```python
from build123d import *

# Parameters (mm, degrees)
BOSS_EXTRUDE1_DEPTH      = 11.85
BOSS_EXTRUDE2_DEPTH      = 2
BOSS_EXTRUDE2_DEPTH_BACK = 13.85
SKETCH2_W                = 7
SKETCH2_H                = 1.8
FILLET1_R                = 6
CUT_EXTRUDE1_DEPTH       = 0.5
CUT_EXTRUDE2_DEPTH       = 0.5
SKETCH6_R                = 2.65
SKETCH6_R_2              = 1.5
CUT_EXTRUDE3_DEPTH       = 10


with BuildPart() as part:
    # Sketch1 → Boss-Extrude1 (new body)
    with BuildSketch(Plane.XY):
        with BuildLine():
            Line((-40, 25.458108108), (-17.056531053, 25.458108108))
            ThreePointArc((-17.056531053, 25.458108108), (-18.352562381, 15.292302634), (-15, 5.608108108))
            Line((-15, 5.608108108), (-40, 5.608108108))
            Line((-40, 5.608108108), (-40, 25.458108108))
        make_face()
    extrude(amount=BOSS_EXTRUDE1_DEPTH)

    # Sketch2 → Boss-Extrude2 (add, two sides: drawn at the far end of the back side and taken through both)
    with BuildSketch(Plane(origin=(0, 0, 0), x_dir=(-1, 0, 0), z_dir=(0, 0, -1)).offset(-BOSS_EXTRUDE2_DEPTH_BACK)):
        with Locations((36.5, 6.508108108)):
            Rectangle(SKETCH2_W, SKETCH2_H)
        with Locations((36.5, 24.558108108)):
            Rectangle(SKETCH2_W, SKETCH2_H)
    extrude(amount=BOSS_EXTRUDE2_DEPTH + BOSS_EXTRUDE2_DEPTH_BACK)

    # Fillet1
    # the kernel refuses this fillet: 6 mm, written as the material it takes off along each edge
    with BuildSketch(Plane(origin=(4, 17.608108108, 0), x_dir=(-0.5195868737353421, 0.854417626598336, 0), z_dir=(0.854417626598336, 0.5195868737353421, 0))) as fillet1_piece_1:
        with BuildLine():
            CenterArc((22.472205054 + FILLET1_R, FILLET1_R), FILLET1_R, 180, 90)
            Line((22.472205054 + FILLET1_R, 0), (22.472205054, 0))
            Line((22.472205054, 0), (22.472205054, FILLET1_R))
        make_face()
    revolve(axis=Axis((4, 17.608108108, 0), (0, 0, 1)), revolution_arc=129.220802233, mode=Mode.SUBTRACT)
    with BuildSketch(Plane(origin=(4, 17.608108108, 11.85), x_dir=(-0.5195868737353421, 0.854417626598336, 0), z_dir=(0.854417626598336, 0.5195868737353421, 0))) as fillet1_piece_2:
        with BuildLine():
            CenterArc((22.472205054 + FILLET1_R, -FILLET1_R), FILLET1_R, 90, 90)
            Line((22.472205054, -FILLET1_R), (22.472205054, 0))
            Line((22.472205054, 0), (22.472205054 + FILLET1_R, 0))
        make_face()
    revolve(axis=Axis((4, 17.608108108, 11.85), (0, 0, 1)), revolution_arc=129.220802233, mode=Mode.SUBTRACT)

    # Sketch3 → Cut-Extrude1 (cut)
    with BuildSketch(Plane(origin=(0, 25.458108108, 0), x_dir=(1, 0, 0), z_dir=(0, 1, 0))):
        with BuildLine():
            Line((-40, -0.925), (-22.180241126, -0.925))
            add(Edge.make_bspline(
                [(-18.937526934, -2.925), (-19.013227922, -2.828512493), (-19.092514949, -2.73433601), (-19.290739716, -2.514692345), (-19.412819443, -2.391961398), (-19.796517456, -2.041181837), (-20.076726357, -1.829898628), (-20.674341708, -1.461904013), (-20.986869841, -1.307747212), (-21.591258811, -1.074971042), (-21.88385471, -0.988046248), (-22.180241126, -0.925)],
                knots=[0.393521627, 0.393521627, 0.393521627, 0.393521627, 0.4375, 0.4375, 0.5, 0.5, 0.625, 0.625, 0.75, 0.75, 0.857744944, 0.857744944, 0.857744944, 0.857744944], degree=3))
            Line((-18.937526934, -2.925), (-40, -2.925))
            Line((-40, -2.925), (-40, -0.925))
        make_face()
        with BuildLine():
            Line((-40, -4.925), (-17.97760602, -4.925))
            add(Edge.make_bspline(
                [(-17.857114262, -5.924996789), (-17.862389732, -5.585330665), (-17.903230985, -5.251628442), (-17.97760602, -4.925)],
                knots=[0, 0, 0, 0, 0.123073848, 0.123073848, 0.123073848, 0.123073848], degree=3))
            add(Edge.make_bspline(
                [(-17.977607618, -6.925), (-17.903108355, -6.597642735), (-17.862351336, -6.26181668), (-17.857114262, -5.924996789)],
                knots=[0.87810057, 0.87810057, 0.87810057, 0.87810057, 1, 1, 1, 1], degree=3))
            Line((-17.977607618, -6.925), (-40, -6.925))
            Line((-40, -6.925), (-40, -4.925))
        make_face()
        with BuildLine():
            Line((-40, -8.925), (-18.937485208, -8.925))
            add(Edge.make_bspline(
                [(-22.180090087, -10.925), (-22.058031588, -10.899076779), (-21.936790659, -10.869159263), (-21.647506804, -10.787627729), (-21.479286663, -10.731759415), (-20.988005272, -10.542973422), (-20.675799804, -10.388674568), (-20.230975304, -10.115240101), (-20.087143687, -10.017400974), (-19.80724707, -9.806950573), (-19.671333831, -9.694234428), (-19.322525279, -9.375728013), (-19.120509969, -9.15842179), (-18.937485208, -8.925)],
                knots=[0.142746843, 0.142746843, 0.142746843, 0.142746843, 0.1875, 0.1875, 0.25, 0.25, 0.375, 0.375, 0.4375, 0.4375, 0.5, 0.5, 0.607411447, 0.607411447, 0.607411447, 0.607411447], degree=3))
            Line((-22.180090087, -10.925), (-40, -10.925))
            Line((-40, -10.925), (-40, -8.925))
        make_face()
    extrude(amount=-CUT_EXTRUDE1_DEPTH, mode=Mode.SUBTRACT)

    # Sketch4 → Cut-Extrude2 (cut)
    with BuildSketch(Plane.XZ.offset(-5.608108108)):
        with BuildLine():
            Line((-18.937485208, 8.925), (-40, 8.925))
            Line((-40, 8.925), (-40, 10.925))
            Line((-40, 10.925), (-22.180090087, 10.925))
            add(Edge.make_bspline(
                [(-22.180090087, 10.925), (-22.058031589, 10.899076779), (-21.936790659, 10.869159263), (-21.647506804, 10.787627729), (-21.479286663, 10.731759415), (-20.988005272, 10.542973422), (-20.675799804, 10.388674568), (-20.230975304, 10.115240101), (-20.087143687, 10.017400974), (-19.80724707, 9.806950573), (-19.671333831, 9.694234428), (-19.322525301, 9.375728033), (-19.12051001, 9.158421833), (-18.937485208, 8.925)],
                knots=[0.392588564, 0.392588564, 0.392588564, 0.392588564, 0.437341721, 0.437341721, 0.499841721, 0.499841721, 0.624841721, 0.624841721, 0.687341721, 0.687341721, 0.749841721, 0.749841721, 0.857253157, 0.857253157, 0.857253157, 0.857253157], degree=3))
        make_face()
        with BuildLine():
            Line((-40, 6.925), (-17.977607618, 6.925))
            add(Edge.make_bspline(
                [(-17.977607618, 6.925), (-17.903108355, 6.597642735), (-17.862351336, 6.26181668), (-17.857114262, 5.924996789)],
                knots=[0, 0, 0, 0, 0.12189943, 0.12189943, 0.12189943, 0.12189943], degree=3))
            add(Edge.make_bspline(
                [(-17.857114262, 5.924996789), (-17.862389732, 5.585330665), (-17.903230985, 5.251628442), (-17.97760602, 4.925)],
                knots=[0.876926152, 0.876926152, 0.876926152, 0.876926152, 1, 1, 1, 1], degree=3))
            Line((-17.97760602, 4.925), (-40, 4.925))
            Line((-40, 4.925), (-40, 6.925))
        make_face()
        with BuildLine():
            Line((-40, 2.925), (-18.937526934, 2.925))
            add(Edge.make_bspline(
                [(-18.937526934, 2.925), (-19.013227922, 2.828512493), (-19.092514949, 2.73433601), (-19.290739716, 2.514692345), (-19.412819443, 2.391961398), (-19.796517456, 2.041181837), (-20.076726357, 1.829898628), (-20.674341708, 1.461904013), (-20.986869841, 1.307747212), (-21.591258789, 1.07497105), (-21.883854665, 0.988046261), (-22.180241126, 0.925)],
                knots=[0.142255064, 0.142255064, 0.142255064, 0.142255064, 0.186233438, 0.186233438, 0.248733438, 0.248733438, 0.373733438, 0.373733438, 0.498733438, 0.498733438, 0.606478373, 0.606478373, 0.606478373, 0.606478373], degree=3))
            Line((-22.180241126, 0.925), (-40, 0.925))
            Line((-40, 0.925), (-40, 2.925))
        make_face()
    extrude(amount=-CUT_EXTRUDE2_DEPTH, mode=Mode.SUBTRACT)

    # Sketch6 → Cut-Extrude3 (cut)
    with BuildSketch(Plane.ZY.offset(40)):
        with Locations((2.85, 15.458108108)):
            Circle(SKETCH6_R)
        with Locations((2.85, 15.458108108)):
            Circle(SKETCH6_R_2, mode=Mode.SUBTRACT)
    extrude(amount=-CUT_EXTRUDE3_DEPTH, mode=Mode.SUBTRACT)


solid = part.part
```
CAD build for the part. Positions are in the model's coordinates, mm. A direction names the side the tool comes from. Give positions to 0.01 mm unless a question says otherwise; leave off trailing zeros. Loops run counter-clockwise (first coordinate to the right, second up) from the corner with the lowest first, then second, coordinate; pieces in that order, holes last. Notation, with made-up numbers: (-25.5, 10.5) -> (2.5, 10.5) arc R9 ccw to (2.5, 16.5) -> close; hole circle Ø9 at (63, -3). An arc over 180 degrees is marked (long way). Use a Markdown table: item, result.
1. Slice it at A-A (x = -28.75). List the corners of the cut face in (y, z) (3 decimals), plus the area to 3 significant figures.
Check result:
| item | result |
|---|---|
| outline | (5.608, 0) -> (25.458, 0) -> (25.458, 0.925) -> (24.958, 0.925) -> (24.958, 2.925) -> (25.458, 2.925) -> (25.458, 4.925) -> (24.958, 4.925) -> (24.958, 6.925) -> (25.458, 6.925) -> (25.458, 8.925) -> (24.958, 8.925) -> (24.958, 10.925) -> (25.458, 10.925) -> (25.458, 11.85) -> (5.608, 11.85) -> (5.608, 10.925) -> (6.108, 10.925) -> (6.108, 8.925) -> (5.608, 8.925) -> (5.608, 6.925) -> (6.108, 6.925) -> (6.108, 4.925) -> (5.608, 4.925) -> (5.608, 2.925) -> (6.108, 2.925) -> (6.108, 0.925) -> (5.608, 0.925) -> close |
| area | 229 mm^2 |
2. Mould opens along Z. For faces 6 (the flat face through (-36, 7, -2)), 7 (the flat face through (-29, 6.108, 10)), 8 (the flat face through (-40, 15, 6)) say: pulls with the +Z half, pulls with the -Z half, needs draft (parallel to the pull), parting line crosses it, or undercut.
Check result:
| item | result |
|---|---|
| face 6 | pulls with the -Z half |
| face 7 | undercut |
| face 8 | needs draft |
3. Slice it at C-C (x = -35.5). Give the number of separate pieces and of enclosed holes in the cut face, plus the area to 3 significant figures.
Check result:
| item | result |
|---|---|
| separate pieces | 2 |
| enclosed holes | 1 |
| area | 229 mm^2 |
4. Flat gauge pins, fed straight in: pin 1 (1.5 mm diameter, centred on x = -25.5, z = 6, fed in from +Y); pin 2 (9 mm diameter, centred on x = -27.5, y = 13, fed in from -Z); pin 3 (6 mm diameter, centred on y = 8, z = 2, fed in from +X); pin 4 (1.6 mm diameter, centred on x = -24, z = 6.5, fed in from +Y). Where does each tip first touch, or does it go through?
Check result:
| item | result |
|---|---|
| pin 1 | stops at y = 24.96 |
| pin 2 | stops at z = 0 |
| pin 3 | stops at x = -15.49 |
| pin 4 | stops at y = 25.46 |
5. Slice it at B-B (z = 0.5). List the corners of the cut face in (x, y).
Check result:
| item | result |
|---|---|
| outline | (-40, 5.61) -> (-19.15, 5.61) arc R26.07 cw to (-20.86, 25.46) -> (-40, 25.46) -> (-40, 16.68) -> (-30, 16.68) -> (-30, 14.23) -> (-40, 14.23) -> close |
6. Which spindle directions (+Z, -Z, +X, -X, +Y, -Y) get a long thin tool onto all of the face, cutting with end or side? Do faces 1 (the flat face through (-33, 25, 13)), 2 (the flat face through (-36, 23.658, -1)), 3 (the cylindrical face through (-35.07, 12.87, 2.28)), 4 (the flat face through (-33, 25, -1)), 5 (the flat face through (-29, 24.958, 6)). Say none if no direction does.
Check result:
| item | result |
|---|---|
| face 1 | +Z, +X, +Y, -Y |
| face 2 | -Z, +X, -X |
| face 3 | -X |
| face 4 | -Z, +X, +Y, -Y |
| face 5 | -X, +Y |
7. Wall check: L1, parallel to Y at x = -37.5, z = 2.85; L2, parallel to Z at x = -36.5, y = 20.5; L3, parallel to X at y = 24, z = -0.25. Give the ranges that are in metal, low to high. Write a range as [from, to].
Check result:
| item | result |
|---|---|
| L1 | y = [6.11, 12.81], [13.96, 16.96], [18.11, 24.96] |
| L2 | z = [0, 11.85] |
| L3 | x = [-40, -33] |
